Input: part model. Units: mm. Frame: model coordinates. Face numbers are marked on the shaded views. A direction names the side the tool comes from. Round coordinates to 2 decimals unless told otherwise and drop trailing zeros. Loops run counter-clockwise (first coordinate to the right, second up) from the corner with the lowest first, then second, coordinate; pieces in that order, holes last. Notation, with made-up numbers: (86.25, -24.5) -> (138.25, -24.5) arc R23 ccw to (138.25, -11.5) -> close; hole circle Ø10 at (57.25, 39). An arc over 180 degrees is marked (long way). Answer in a Markdown table with one row per item. Add a question column.
Q1. Section B-B, the plane z = 105. Output: boundary loops of the cut face in (x, y), and give its area (3 significant figures).
Q2. Reachability of the marked faces 1 and 2 from +Z, -Z, +X, -X, +Y, -Y: full face, straight path, thin tool, end or side. Return the list, or none.
Q3. Ray query, L1, parallel to Z at x = 58.5, y = 6; L2, parallel to Y at x = 73, z = 230; L3, parallel to Z at x = 141, y = 8.5. Return the intervals inside material, ascending. Write a range as from..to.
Q4. Section C-C, the plane x = 9. Output: boundary loops of the cut face in (y, z).
Q5. Section A-A, the plane x = 43.5. Output: boundary loops of the cut face in (y, z) (3 decimals).
Q6. Pin query (flat end, axial travel): pin 1 (6 mm diameter, centred on x = 63, z = 144.5, fed in from -Y); pin 2 (3.5 mm diameter, centred on x = 64, y = 6, fed in from -Z); pin 3 (1.1 mm diameter, centred on y = 0, z = 0, fed in from -X); pin 4 (3 mm diameter, centred on x = 30.5, y = -2.5, fed in from +Z). Return the tip coordinate at first contact, or that it passes through.
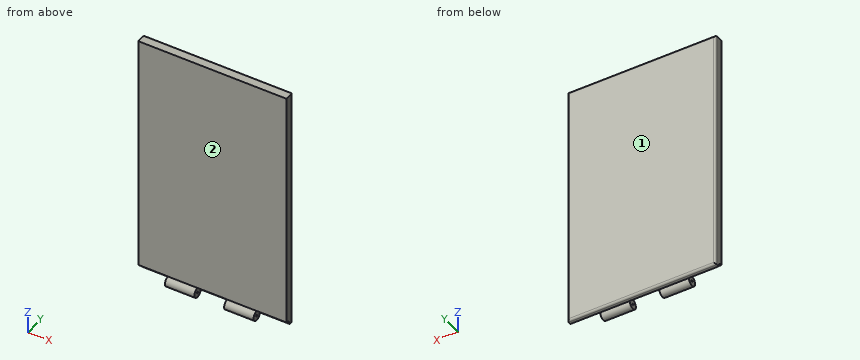
```python
from build123d import *

# Parameters (mm, degrees)
SKETCH1_W           = 150
SKETCH1_H           = 10
BOSS_EXTRUDE1_DEPTH = 250
FILLET1_R           = 2
SKETCH2_R           = 5.1
CUT_EXTRUDE1_DEPTH  = 30.1
SKETCH3_R           = 5
BOSS_EXTRUDE2_DEPTH = 29.85
SKETCH4_R           = 5.1
CUT_EXTRUDE2_DEPTH  = 30.1
SKETCH5_R           = 5
BOSS_EXTRUDE3_DEPTH = 29.85
SKETCH6_R           = 5.1
CUT_EXTRUDE3_DEPTH  = 30.1
SKETCH7_R           = 0.875
CUT_EXTRUDE4_DEPTH  = 90.1


with BuildPart() as part:
    # Sketch1 → Boss-Extrude1 (new body)
    with BuildSketch(Plane.XY):
        with Locations((75, 5)):
            Rectangle(SKETCH1_W, SKETCH1_H)
    extrude(amount=BOSS_EXTRUDE1_DEPTH)

    # Fillet1
    fillet1_edges = [part.edges().sort_by_distance(p)[0] for p in [
        (75, 10, 250),
        (75, 10, 0),
        (0, 10, 125),
        (150, 10, 125),
    ]]
    fillet(fillet1_edges, radius=FILLET1_R)

    # Sketch2 → Cut-Extrude1 (cut)
    with BuildSketch(Plane(origin=(150, 0, 0), x_dir=(0, 0, -1), z_dir=(1, 0, 0))):
        Circle(SKETCH2_R)
    extrude(amount=-CUT_EXTRUDE1_DEPTH, mode=Mode.SUBTRACT)

    # Sketch3 → Boss-Extrude2 (add)
    with BuildSketch(Plane(origin=(119.9, 0, 0), x_dir=(0, 0, -1), z_dir=(1, 0, 0))):
        Circle(SKETCH3_R)
    extrude(amount=-BOSS_EXTRUDE2_DEPTH)

    # Sketch4 → Cut-Extrude2 (cut)
    with BuildSketch(Plane.ZY.offset(-90.05)):
        Circle(SKETCH4_R)
    extrude(amount=CUT_EXTRUDE2_DEPTH, mode=Mode.SUBTRACT)

    # Sketch5 → Boss-Extrude3 (add)
    with BuildSketch(Plane(origin=(59.95, 0, 0), x_dir=(0, 0, -1), z_dir=(1, 0, 0))):
        Circle(SKETCH5_R)
    extrude(amount=-BOSS_EXTRUDE3_DEPTH)

    # Sketch6 → Cut-Extrude3 (cut)
    with BuildSketch(Plane.ZY.offset(-30.1)):
        Circle(SKETCH6_R)
    extrude(amount=CUT_EXTRUDE3_DEPTH, mode=Mode.SUBTRACT)

    # Sketch7 → Cut-Extrude4 (cut)
    with BuildSketch(Plane(origin=(119.9, 0, 0), x_dir=(0, 0, -1), z_dir=(1, 0, 0))):
        Circle(SKETCH7_R)
    extrude(amount=-CUT_EXTRUDE4_DEPTH, mode=Mode.SUBTRACT)


solid = part.part
```
Answer block:
| question | item | result |
|---|---|---|
| 1 | outline | (0, 0) -> (150, 0) -> (150, 8) arc R2 ccw to (148, 10) -> (2, 10) arc R2 ccw to (0, 8) -> close |
| 1 | area | 1,500 mm^2 |
| 2 | face 1 | +Z, -Z, +X, -X, +Y |
| 2 | face 2 | +Z, +X, -X, -Y |
| 3 | L1 | 0..250 |
| 3 | L2 | 0..10 |
| 3 | L3 | 0.06..249.94 |
| 4 | outline | (0, 5.1) arc R5.1 cw to (5.1, 0) -> (8, 0) arc R2 ccw to (10, 2) -> (10, 248) arc R2 ccw to (8, 250) -> (0, 250) -> close |
| 5 | outline | (0, 5) arc R5 ccw (long way) to (5, 0) -> (8, 0) arc R2 ccw to (10, 2) -> (10, 248) arc R2 ccw to (8, 250) -> (0, 250) -> close; hole circle Ø1.75 at (0, 0) |
| 6 | pin 1 | y = 0 |
| 6 | pin 2 | z = 0 |
| 6 | pin 3 | through |
| 6 | pin 4 | z = 4.9 |
